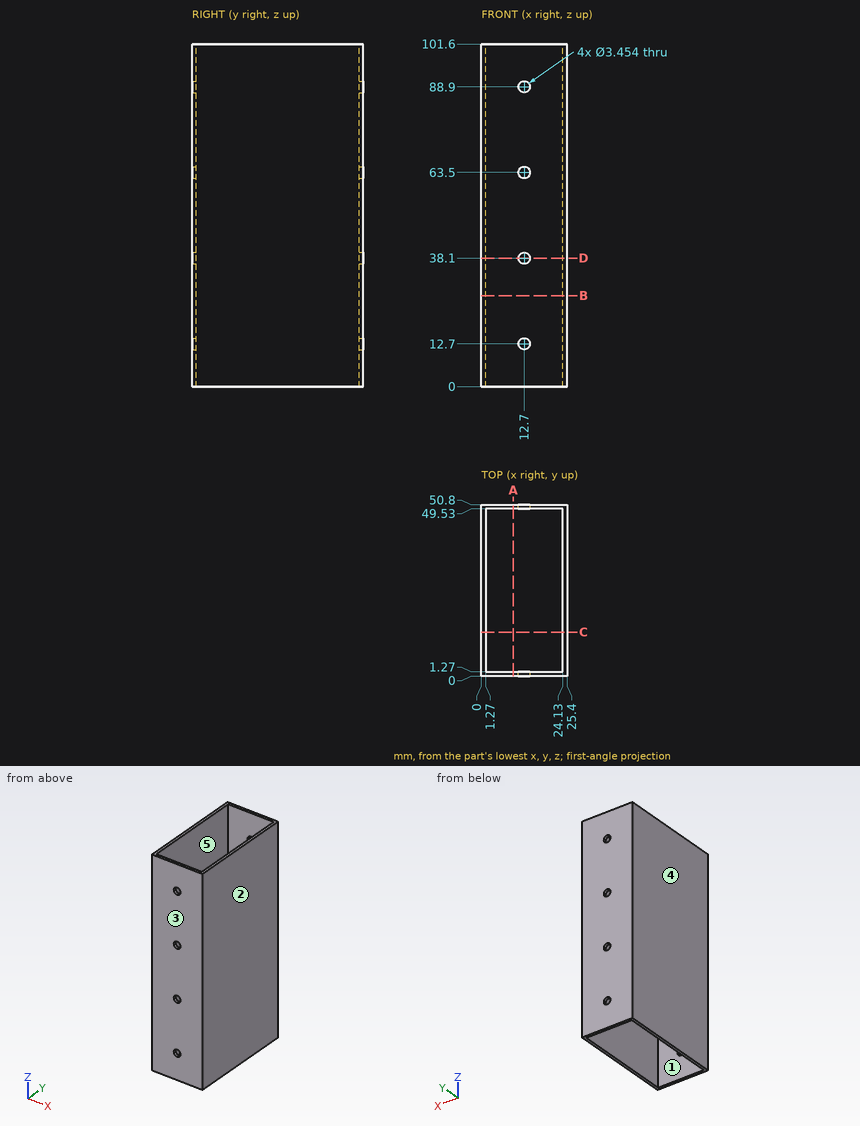
Geometry check sheet. Reference: drawing and pictorial views, mm from the part's lowest x, y, z. A direction names the side the tool comes from. Give positions to 0.01 mm unless a question says otherwise; leave off trailing zeros. Order: outer loops, then holes, each group sorted by start corner. A loop starts at its lowest first (then second) coordinate and runs counter-clockwise, first axis right, second up. Notation, with made-up numbers: M -4,40.5 L 34,40.5 A18 ccw 34,61.5 Z; hole C 26,46 d6. An arc over 180 degrees is marked long. Answer in a Markdown table with one row per item.
1) Gauge pin test, flat end, axial feed: P1, Ø3, axis at x = 12.7, z = 63.5, coming from the +Y side. Record the tip position at first contact, or that the pin passes through.
Filled sheet:
| item | result |
|---|---|
| P1 | passes through |
2) Thickness scan on L1, parallel to Z at x = 12.7, y = 50.5; L2, parallel to Y at x = 3, z = 90; L3, parallel to X at y = 37.5, z = 65. Record the ranges inside material, lowest first. Write a range as [from, to].
Filled sheet:
| item | result |
|---|---|
| L1 | z = [0, 10.97], [14.43, 36.37], [39.83, 61.77], [65.23, 87.17], [90.63, 101.6] |
| L2 | y = [0, 1.27], [49.53, 50.8] |
| L3 | x = [0, 1.27], [24.13, 25.4] |
3) Access from +Z, -Z, +X, -X, +Y, -Y to the whole of each face (thin tool, end or side, straight path). Record for the marked faces 4 and 5.
Filled sheet:
| item | result |
|---|---|
| face 4 | +Z, -Z, -X, +Y, -Y |
| face 5 | +Z, -Z |
4) Cross-section at A-A, the plane x = 9.5. Enter the section's corners in (y, z), plus the area to 3 significant figures.
Filled sheet:
| item | result |
|---|---|
| outline | M 0,0 L 1.27,0 L 1.27,101.6 L 0,101.6 Z; M 49.53,0 L 50.8,0 L 50.8,101.6 L 49.53,101.6 Z |
| area | 258 mm2 |
5) Cross-section at B-B, the plane z = 27. Enter the section's corners in (x, y).
Filled sheet:
| item | result |
|---|---|
| outline | M 0,0 L 25.4,0 L 25.4,50.8 L 0,50.8 Z; hole M 1.27,1.27 L 24.13,1.27 L 24.13,49.53 L 1.27,49.53 Z |
6) Cross-section at C-C, the plane y = 13. Enter the section's corners in (x, z).
Filled sheet:
| item | result |
|---|---|
| outline | M 0,0 L 1.27,0 L 1.27,101.6 L 0,101.6 Z; M 24.13,0 L 25.4,0 L 25.4,101.6 L 24.13,101.6 Z |
7) Release check for a two-part mould opening along X. For the marked faces 1, 2 and 3 record: +X half, -X half, draft (parallel to the pull), parting line (faces both ways), or undercut.
Filled sheet:
| item | result |
|---|---|
| face 1 | undercut |
| face 2 | +X half |
| face 3 | draft |
8) Cross-section at D-D, the plane z = 38.1. Enter the section's corners in (x, y).
Filled sheet:
| item | result |
|---|---|
| outline | M 0,0 L 10.97,0 L 10.97,1.27 L 1.27,1.27 L 1.27,49.53 L 10.97,49.53 L 10.97,50.8 L 0,50.8 Z; M 14.43,0 L 25.4,0 L 25.4,50.8 L 14.43,50.8 L 14.43,49.53 L 24.13,49.53 L 24.13,1.27 L 14.43,1.27 Z |
